Answer from the drawing. Dimensions are ordinates in mm from the lowest x, y and z of the part. A direction names the side the tool comes from. Give positions to 0.01 mm unless a question says otherwise; leave off trailing zeros. Order: outer loops, then holes, each group sorted by start corner. A loop starts at its lowest first (then second) coordinate and runs counter-clockwise, first axis right, second up. Notation, with made-up numbers: M 56,-38 L 90,-38 A19 ccw 90,-9 Z; hole C 86,-17 d6. An arc over 180 degrees is marked long. One line per item, written item: value.
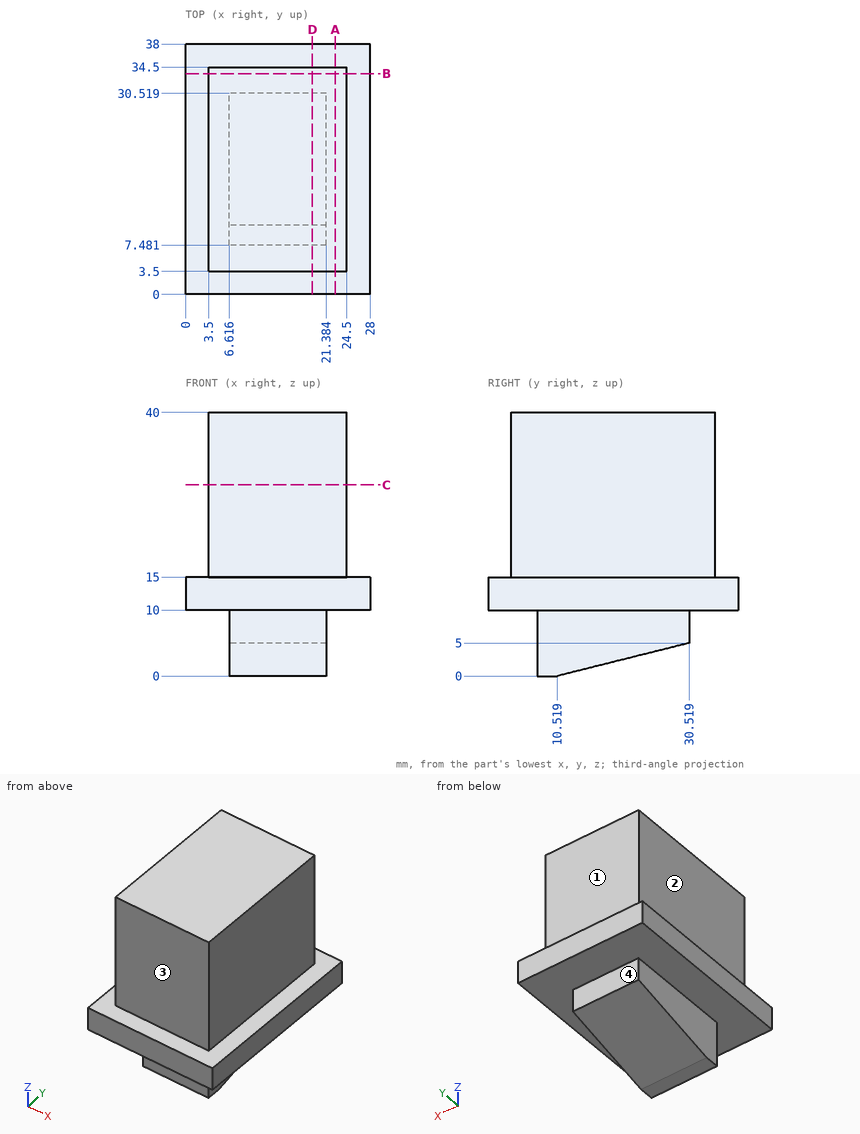
(1) Section C-C, the plane z = 29 is taken. Give the vertices of the cut face in (x, y), then the cut area to 3 significant figures.
Findings:
outline: M 3.5,3.5 L 24.5,3.5 L 24.5,34.5 L 3.5,34.5 Z
area: 651 mm^2
(2) Given P1, Ø6, axis at x = 13.5, y = 12, coming from the -Z side; P2, Ø20, axis at y = 24, z = 31, coming from the +X side; P3, Ø2, axis at x = 7.5, z = 19, coming from the -Y side; P4, Ø7.5, axis at y = 12, z = 30.5, coming from the -X side, each flat-ended and moving along its own axis, determine where each tip first touches the part or whether it passes through.
Findings:
P1: stops at z = 0
P2: stops at x = 24.5
P3: stops at y = 3.5
P4: stops at x = 3.5
(3) Section D-D, the plane x = 19.25 is taken. Give the vertices of the cut face in (y, z).
Findings:
outline: M 0,10 L 7.48,10 L 7.48,0 L 10.52,0 L 30.52,5 L 30.52,10 L 38,10 L 38,15 L 34.5,15 L 34.5,40 L 3.5,40 L 3.5,15 L 0,15 Z
(4) Which of the six approach directions +Z, -Z, +X, -X, +Y, -Y give full straight-line access (tool end or side, diameter ignored) to the marked faces 1, 2, 3 and 4?
Findings:
face 1: +Z, +X, -X, +Y
face 2: +Z, -X, +Y, -Y
face 3: +Z, +X, -X, -Y
face 4: -Z, +X, -X, +Y
(5) Section B-B, the plane y = 33.5 is taken. Give the vertices of the cut face in (x, z).
Findings:
outline: M 0,10 L 28,10 L 28,15 L 24.5,15 L 24.5,40 L 3.5,40 L 3.5,15 L 0,15 Z
(6) Find the intervals of material crossed by probe 1 along X at (y, z) = (31, 30); probe 2 along Z at (x, y) = (24.75, 16); probe 3 along Y at (x, z) = (16.5, 8.5), in increasing order. Write a range as from..to.
Findings:
probe 1: x = 3.5..24.5
probe 2: z = 10..15
probe 3: y = 7.48..30.52
(7) Section A-A, the plane x = 22.75 is taken. Give the vertices of the cut face in (y, z), then the cut area to 3 significant figures.
Findings:
outline: M 0,10 L 38,10 L 38,15 L 34.5,15 L 34.5,40 L 3.5,40 L 3.5,15 L 0,15 Z
area: 965 mm^2
